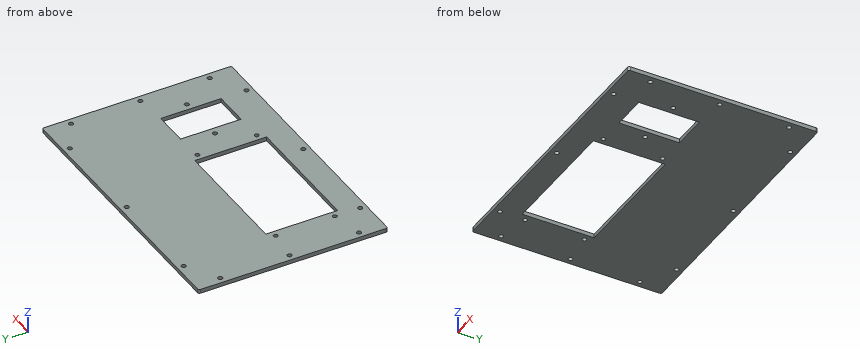
```python
from build123d import *

# Parameters (mm, degrees)
SKETCH1_W            = 220
SKETCH1_H            = 150
BOSS_EXTRUDE1_DEPTH  = 3.175
M3_CLEARANCE_HOLE1_D = 3.6
SKETCH4_W            = 10
SKETCH4_H            = 10
BOSS_EXTRUDE2_DEPTH  = 3.175
FILLET2_R            = 1.5
SKETCH5_W            = 28
SKETCH5_H            = 48
CUT_EXTRUDE1_DEPTH   = 4.175
M3_CLEARANCE_HOLE2_D = 3.6
SKETCH8_W            = 100
SKETCH8_H            = 57
CUT_EXTRUDE2_DEPTH   = 4.175
M3_CLEARANCE_HOLE3_D = 3.4


with BuildPart() as part:
    # Sketch1 → Boss-Extrude1 (new body)
    with BuildSketch(Plane.XY):
        Rectangle(SKETCH1_W, SKETCH1_H)
    extrude(amount=BOSS_EXTRUDE1_DEPTH)

    # M3 Clearance Hole1 (through all)
    with Locations(Plane.XY.offset(3.175)):
        with Locations((0, 0), (-80, 70), (80, 70), (0, 70), (-105, 55), (-105, 0), (-105, -55), (-80, -70), (0, -70), (80, -70), (105, -55), (105, 0), (105, 55)):
            Hole(M3_CLEARANCE_HOLE1_D / 2)

    # Sketch4 → Boss-Extrude2 (add, through all)
    with BuildSketch(Plane.XY.offset(3.175)):
        Rectangle(SKETCH4_W, SKETCH4_H)
    extrude(amount=-BOSS_EXTRUDE2_DEPTH)

    # Fillet2
    fillet2_edges = [part.edges().sort_by_distance(p)[0] for p in [
        (-110, -75, 1.5875),
        (-110, 75, 1.5875),
        (110, 75, 1.5875),
        (110, -75, 1.5875),
    ]]
    fillet(fillet2_edges, radius=FILLET2_R)

    # Sketch5 → Cut-Extrude1 (cut, through all)
    with BuildSketch(Plane.XY.offset(3.175)):
        with Locations((66, -26)):
            Rectangle(SKETCH5_W, SKETCH5_H)
    extrude(amount=-CUT_EXTRUDE1_DEPTH, mode=Mode.SUBTRACT)

    # M3 Clearance Hole2 (through all)
    with Locations(Plane.XY.offset(3.175)):
        with Locations((46.25, -26), (85.75, -26)):
            Hole(M3_CLEARANCE_HOLE2_D / 2)

    # Sketch8 → Cut-Extrude2 (cut, through all)
    with BuildSketch(Plane.XY.offset(3.175)):
        with Locations((-25, -26.5)):
            Rectangle(SKETCH8_W, SKETCH8_H)
    extrude(amount=-CUT_EXTRUDE2_DEPTH, mode=Mode.SUBTRACT)

    # M3 Clearance Hole3 (through all)
    with Locations(Plane.XY.offset(3.175)):
        with Locations((-80, -3), (-80, -50), (30, -50), (30, -3)):
            Hole(M3_CLEARANCE_HOLE3_D / 2)


solid = part.part
```
Input: part model. Units: mm. Frame: model coordinates. Round coordinates to 2 decimals unless told otherwise and drop trailing zeros. Order: outer loops, then holes, each group sorted by start corner. A loop starts at its lowest first (then second) coordinate and runs counter-clockwise, first axis right, second up. Notation, with made-up numbers: (-24, -4.75) - (-15, -4.75) arc R17 ccw to (-15, 23.25) - close; hole circle Ø5 at (55, 44). An arc over 180 degrees is marked (long way). Answer in a Markdown table with one row per item.
Item 1: Line query: line 1 (X direction, y = -70, z = 1.8); line 2 (X direction, y = -6, z = 1.6); line 3 (Y direction, x = 105, z = 1.4). Output: solid intervals per line, ascending.
Model answer:
| item | result |
|---|---|
| line 1 | x = -110 to -81.8, -78.2 to -1.8, 1.8 to 78.2, 81.8 to 110 |
| line 2 | x = -110 to -75, 25 to 52, 80 to 110 |
| line 3 | y = -75 to -56.8, -53.2 to -1.8, 1.8 to 53.2, 56.8 to 75 |
Item 2: Section query A-A (z = 2.2). Give the number of separate pieces and of enclosed holes in the cut face, then the cut area to 3 significant figures.
Model answer:
| item | result |
|---|---|
| separate pieces | 1 |
| enclosed holes | 20 |
| area | 25,800 mm² |
Item 3: Section query C-C (y = -34.5). Return the cut outline in (x, z) (3 decimals), then the cut area to 3 significant figures.
Model answer:
| item | result |
|---|---|
| outline | (-110, 0) - (-75, 0) - (-75, 3.175) - (-110, 3.175) - close; (25, 0) - (52, 0) - (52, 3.175) - (25, 3.175) - close; (80, 0) - (110, 0) - (110, 3.175) - (80, 3.175) - close |
| area | 292 mm² |
Item 4: Section query B-B (x = -53). Return the cut outline in (y, z) (3 decimals).
Model answer:
| item | result |
|---|---|
| outline | (-75, 0) - (-55, 0) - (-55, 3.175) - (-75, 3.175) - close; (2, 0) - (75, 0) - (75, 3.175) - (2, 3.175) - close |
